Could you check a few things on this model? Use its own coordinates, in mm. A direction names the side the tool comes from. Give positions to 0.01 mm unless a question says otherwise; leave off trailing zeros. Write each loop counter-clockwise with the first axis right and the second up, starting at its lowest first coordinate (ties: lowest second). Pieces come first, ordered by that corner, then holes. Notation, with made-up numbers: (61.5, 75.25) - (109.5, 75.25) arc R21 ccw to (109.5, 89.25) - close; hole circle Ø10 at (7, -25). An arc over 180 degrees is marked (long way). Answer as CSV lines item,"result". Start each with the question number.
Q1. Imagine slicing it at A-A on z = 2. State how many separate pieces and enclosed holes the cut face has, and give its area (3 significant figures).
Q2. We'd pull the mould along X, two halves only. Please class faces 1 (the face through (-4, 10, 2)), 2 (the face through (-3.3, -19.57, 2.51)), 3 (the face through (-5, 0, 2)): pulls with the +X half, pulls with the -X half, needs draft (parallel to the pull), parting line crosses it, or undercut.
Q3. Imagine slicing it at B-B on x = 0.5. List the corners of the cut face in (y, z) for me, and give its area (3 significant figures).
Q4. On a 3-axis mill with a long thin cutter (end or side, diameter ignored), from which of +Z, -Z, +X, -X, +Y, -Y can I reach the whole of each face in a straight line? I mean faces 4 (the face through (0, 20, 2)), 5 (the face through (0, -19, 2)). Say none if no direction works.
Q5. If I drill on line 1 along Y through (x, z) = (-1.5, 1.3); line 2 along Z through (x, y) = (-2.75, 19.55); line 3 along X through (y, z) = (10, 2.1), over which ranges is the centre line in solid material (lowest first)?
Q6. Imagine slicing it at C-C on z = 3.5. List the corners of the cut face in (x, y) for me.
Q7. Imagine slicing it at D-D on y = 13. List the corners of the cut face in (x, z) for me.
Q8. Will this pin go through, and if not, where does the flat tip stop? pin 1 Ø1.2 at (y, z) = (-10, 1.5) entering from +X.
```python
from build123d import *

# Parameters (mm, degrees)
F2_W     = 10
F2_H     = 40
F3_DEPTH = 4
F4_W     = 9
F4_H     = 18.5
F5_DEPTH = 4.001
F6_R     = 0.75
F7_DEPTH = 40.001
F8_R     = 0.125


with BuildPart() as f3:
    # F2 (on Top) → F3 (new body)
    with BuildSketch(Plane.XY):
        Rectangle(F2_W, F2_H)
    extrude(amount=F3_DEPTH)

    # F4 (on face) → F5 (cut, through all)
    with BuildSketch(Plane.XY.offset(4)):
        with Locations((0.5, 9.75)):
            Rectangle(F4_W, F4_H)
        with Locations((0.5, -9.75)):
            Rectangle(F4_W, F4_H)
    extrude(amount=-F5_DEPTH, mode=Mode.SUBTRACT)

    # F6 (on face) → F7 (cut, through all)
    with BuildSketch(Plane.XZ.offset(20)):
        with Locations((-2.75, 2)):
            Circle(F6_R)
    extrude(amount=-F7_DEPTH, mode=Mode.SUBTRACT)

    # F8
    f8_edges = [f3.edges().sort_by_distance(p)[0] for p in [
        (-3.5, -19, 2),
        (-3.5, -0.5, 2),
        (-3.5, 19, 2),
        (-3.5, 0.5, 2),
    ]]
    fillet(f8_edges, radius=F8_R)


solid = f3.part
```
Conclusion:
1,separate pieces,"4"
1,enclosed holes,"0"
1,area,"62.5 mm^2"
2,face 1,"pulls with the +X half"
2,face 2,"undercut"
2,face 3,"pulls with the -X half"
3,outline,"(-20, 0) - (-19, 0) - (-19, 4) - (-20, 4) - close; (-0.5, 0) - (0.5, 0) - (0.5, 4) - (-0.5, 4) - close; (19, 0) - (20, 0) - (20, 4) - (19, 4) - close"
3,area,"12.0 mm^2"
4,face 4,"+Z, -Z, +X, -X, +Y"
4,face 5,"+Z, -Z, +X"
5,line 1,"-20 to -19, -0.5 to 0.5, 19 to 20"
5,line 2,"0 to 1.25, 2.75 to 4"
5,line 3,"-5 to -4"
6,outline,"(-5, -20) - (5, -20) - (5, -19) - (-4, -19) - (-4, -0.5) - (5, -0.5) - (5, 0.5) - (-4, 0.5) - (-4, 19) - (5, 19) - (5, 20) - (-5, 20) - close"
7,outline,"(-5, 0) - (-4, 0) - (-4, 4) - (-5, 4) - close"
8,pin 1,"x = -4"
